The listing builds one solid part. Answer for the finished solid, in the listing's coordinates (mm). A direction names the side the tool comes from. Coordinates: 2 decimals unless noted, no trailing zeros. Write each loop counter-clockwise with the first axis right and the second up, starting at its lowest first coordinate (ties: lowest second). Pieces come first, ordered by that corner, then holes.
from build123d import *

# Parameters (mm, degrees)
SKETCH1_W           = 88.9
SKETCH1_H           = 88.9
BOSS_EXTRUDE1_DEPTH = 5
SKETCH2_R           = 34
BOSS_EXTRUDE2_DEPTH = 6
SKETCH3_W           = 20
SKETCH3_H           = 15
BOSS_EXTRUDE3_DEPTH = 5
SKETCH4_R           = 3.25
CUT_EXTRUDE1_DEPTH  = 5
FILLET1_R           = 15
FILLET2_R           = 5


with BuildPart() as part:
    # Sketch1 → Boss-Extrude1 (new body)
    with BuildSketch(Plane(origin=(0, 0, 0), x_dir=(1, 0, 0), z_dir=(0, 1, 0))):
        Rectangle(SKETCH1_W, SKETCH1_H)
    extrude(amount=BOSS_EXTRUDE1_DEPTH)

    # Sketch2 → Boss-Extrude2 (add)
    with BuildSketch(Plane(origin=(0, 5, 0), x_dir=(1, 0, 0), z_dir=(0, 1, 0))):
        with Locations(Location((0, 0, 0), (0, 0, 270))):
            Circle(SKETCH2_R)
    extrude(amount=BOSS_EXTRUDE2_DEPTH)

    # Sketch3 → Boss-Extrude3 (add)
    with BuildSketch(Plane.XZ):
        with Locations((-10, 51.95)):
            Rectangle(SKETCH3_W, SKETCH3_H)
        with Locations((10, 51.95)):
            Rectangle(SKETCH3_W, SKETCH3_H)
        with Locations((10, -51.95)):
            Rectangle(SKETCH3_W, SKETCH3_H)
        with Locations((-10, -51.95)):
            Rectangle(SKETCH3_W, SKETCH3_H)
    extrude(amount=-BOSS_EXTRUDE3_DEPTH)

    # Sketch4 → Cut-Extrude1 (cut)
    with BuildSketch(Plane.XZ):
        with Locations(Location((10, 51.95, 0), (0, 0, 270))):
            Circle(SKETCH4_R)
        with Locations(Location((-10, 51.95, 0), (0, 0, 270))):
            Circle(SKETCH4_R)
        with Locations(Location((10, -51.95, 0), (0, 0, 270))):
            Circle(SKETCH4_R)
        with Locations(Location((-10, -51.95, 0), (0, 0, 270))):
            Circle(SKETCH4_R)
    extrude(amount=-CUT_EXTRUDE1_DEPTH, mode=Mode.SUBTRACT)

    # Fillet1
    fillet1_edges = [part.edges().sort_by_distance(p)[0] for p in [
        (44.45, 2.5, 44.45),
        (-44.45, 2.5, 44.45),
        (-44.45, 2.5, -44.45),
        (44.45, 2.5, -44.45),
    ]]
    fillet(fillet1_edges, radius=FILLET1_R)

    # Fillet2
    fillet2_edges = [part.edges().sort_by_distance(p)[0] for p in [
        (-20, 2.5, 44.45),
        (-20, 2.5, 59.45),
        (20, 2.5, 59.45),
        (20, 2.5, 44.45),
        (20, 2.5, -44.45),
        (20, 2.5, -59.45),
        (-20, 2.5, -59.45),
        (-20, 2.5, -44.45),
    ]]
    fillet(fillet2_edges, radius=FILLET2_R)


solid = part.part
1. A tool of negligible diameter and unlimited length cuts with its end or side. For faces 1 (the flat face through (39, 5, -1)), 2 (the flat face through (20, 2, 52)), 3 (the cylindrical face through (-21.5, 2.54, -45.88)), from which of +Z, -Z, +X, -X, +Y, -Y can it reach the whole face along a straight path? Write none if from no direction.
Results found:
face 1: +Y
face 2: +Z, +X, +Y, -Y
face 3: -Z, -X, +Y, -Y
2. Flat-ended cylindrical pins translate along their axes: P1, Ø6, axis at y = 4.5, z = -34.5, coming from the -X side; P2, Ø4, axis at y = 1.5, z = -51.5, coming from the -X side; P3, Ø5, axis at x = 19, y = 8, coming from the -Z side. Find the tip coordinate at first contact, or state that the pin passes through.
Results found:
P1: stops at x = -44.31
P2: stops at x = -20
P3: stops at z = -29.73
3. Section C-C on x = -10 is taken. Give the vertices of the cut face in (y, z), then the cut area to 3 significant figures.
Results found:
outline: (0, -59.45) - (5, -59.45) - (5, -55.2) - (0, -55.2) - close; (0, -48.7) - (5, -48.7) - (5, -32.5) - (11, -32.5) - (11, 32.5) - (5, 32.5) - (5, 48.7) - (0, 48.7) - close; (0, 55.2) - (5, 55.2) - (5, 59.45) - (0, 59.45) - close
area: 919 mm2
4. Section D-D on z = 0 is taken. Give the vertices of the cut face in (x, y).
Results found:
outline: (-44.45, 0) - (44.45, 0) - (44.45, 5) - (34, 5) - (34, 11) - (-34, 11) - (-34, 5) - (-44.45, 5) - close
5. For a pull along X with two mould halves and no side action, classify faces 4 (the cylindrical face through (10.98, 2.46, 48.85)), 5 (the cylindrical face through (33.71, 7.96, -4.43)), 6 (the flat face through (0, 2, 59.45)) as pulls with the +X half, pulls with the -X half, needs draft (parallel to the pull), parting line crosses it, or undercut.
Results found:
face 4: undercut
face 5: parting line crosses it
face 6: needs draft
6. Section A-A on z = -51.95 is taken. Give the vertices of the cut face in (x, y), then the cut area to 3 significant figures.
Results found:
outline: (-20, 0) - (-13.25, 0) - (-13.25, 5) - (-20, 5) - close; (-6.75, 0) - (6.75, 0) - (6.75, 5) - (-6.75, 5) - close; (13.25, 0) - (20, 0) - (20, 5) - (13.25, 5) - close
area: 135 mm2
7. Section B-B on y = 2.75 is taken. Give the vertices of the cut face in (x, z), then the cut area to 3 significant figures.
Results found:
outline: (-44.45, -29.45) arc R15 ccw to (-29.45, -44.45) - (-25, -44.45) arc R5 cw to (-20, -49.45) - (-20, -54.45) arc R5 ccw to (-15, -59.45) - (15, -59.45) arc R5 ccw to (20, -54.45) - (20, -49.45) arc R5 cw to (25, -44.45) - (29.45, -44.45) arc R15 ccw to (44.45, -29.45) - (44.45, 29.45) arc R15 ccw to (29.45, 44.45) - (25, 44.45) arc R5 cw to (20, 49.45) - (20, 54.45) arc R5 ccw to (15, 59.45) - (-15, 59.45) arc R5 ccw to (-20, 54.45) - (-20, 49.45) arc R5 cw to (-25, 44.45) - (-29.45, 44.45) arc R15 ccw to (-44.45, 29.45) - close; hole circle Ø6.5 at (-10, -51.95); hole circle Ø6.5 at (-10, 51.95); hole circle Ø6.5 at (10, -51.95); hole circle Ø6.5 at (10, 51.95)
area: 8,780 mm2
8. Find the intervals of material crossed by L1, parallel to X at y = 2.7, z = 51.95; L2, parallel to Y at x = -36.5, z = 7; L3, parallel to Z at x = 26.5, y = 6.25, in increasing order.
Results found:
L1: x = -20 to -13.25, -6.75 to 6.75, 13.25 to 20
L2: y = 0 to 5
L3: z = -21.3 to 21.3
